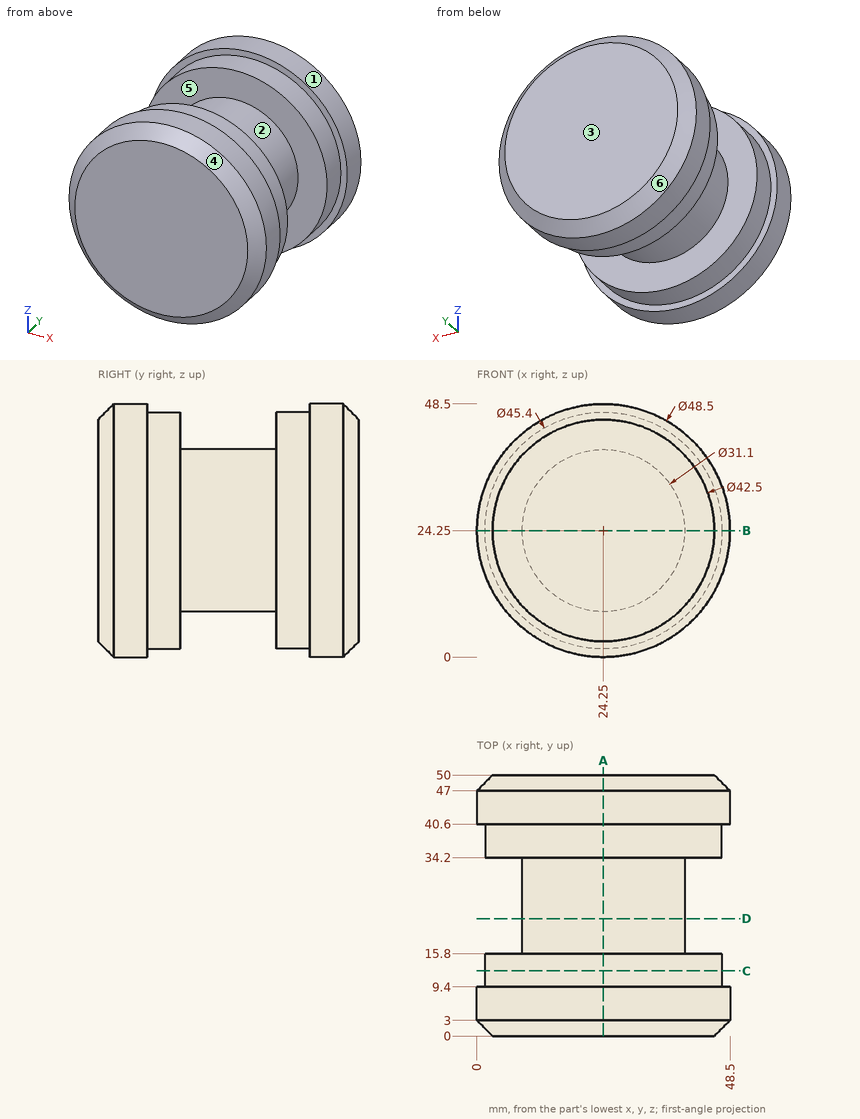
Answer from the drawing. Dimensions are ordinates in mm from the lowest x, y and z of the part. A direction names the side the tool comes from. Coordinates: 2 decimals unless noted, no trailing zeros. Write each loop counter-clockwise with the first axis right and the second up, starting at its lowest first coordinate (ties: lowest second). Pieces come first, ordered by that corner, then holes. Notation, with made-up numbers: (57.25, -14) -> (64.25, -14) arc R23 ccw to (64.25, 21) -> close; hole circle Ø11 at (-17, 40). An arc over 180 degrees is marked (long way). One line per question, with ' | ' between items.
1. Section A-A (x = 24.25) is taken. Determine the outline of the cut face in (y, z), and give its area (3 significant figures).
Verdict:
outline: (0, 3) -> (3, 0) -> (9.4, 0) -> (9.4, 1.55) -> (15.8, 1.55) -> (15.8, 8.7) -> (34.2, 8.7) -> (34.2, 1.55) -> (40.6, 1.55) -> (40.6, 0) -> (47, 0) -> (50, 3) -> (50, 45.5) -> (47, 48.5) -> (40.6, 48.5) -> (40.6, 46.95) -> (34.2, 46.95) -> (34.2, 39.8) -> (15.8, 39.8) -> (15.8, 46.95) -> (9.4, 46.95) -> (9.4, 48.5) -> (3, 48.5) -> (0, 45.5) -> close | area: 2,050 mm^2
2. Given pin 1 Ø2 at (y, z) = (39.5, 22) entering from +X; pin 2 Ø5 at (x, y) = (40.5, 10) entering from +Z; pin 3 Ø4 at (y, z) = (18.5, 31.5) entering from -X, each flat-ended and moving along its own axis, determine where each tip first touches the part or whether it passes through.
Verdict:
pin 1: stops at x = 46.92 | pin 2: stops at z = 44.17 | pin 3: stops at x = 9.61
3. Which of the six approach directions +Z, -Z, +X, -X, +Y, -Y give full straight-line access (tool end or side, diameter ignored) to the marked faces 5 and 6?
Verdict:
face 5: none | face 6: +Y
4. Section D-D (y = 22.5) is taken. Determine the outline of the cut face in (x, z), and give its area (3 significant figures).
Verdict:
outline: circle Ø31.1 at (24.25, 24.25) | area: 760 mm^2
5. Section C-C (y = 12.5) is taken. Determine the outline of the cut face in (x, z).
Verdict:
outline: circle Ø45.4 at (24.25, 24.25)
6. Straight lines are drawn through the part: line 1 (Y direction, x = 7.5, z = 36.5); line 2 (Y direction, x = 23.5, z = 46.5); line 3 (X direction, y = 41, z = 23.5). For each, find the intervals that lie inside material, in ascending order.
Verdict:
line 1: y = 0 to 15.8, 34.2 to 50 | line 2: y = 1.01 to 15.8, 34.2 to 48.99 | line 3: x = 0.01 to 48.49
7. Section B-B (z = 24.25) is taken. Determine the outline of the cut face in (x, y), and give its area (3 significant figures).
Verdict:
outline: (0, 3) -> (3, 0) -> (45.5, 0) -> (48.5, 3) -> (48.5, 9.4) -> (46.95, 9.4) -> (46.95, 15.8) -> (39.8, 15.8) -> (39.8, 34.2) -> (46.95, 34.2) -> (46.95, 40.6) -> (48.5, 40.6) -> (48.5, 47) -> (45.5, 50) -> (3, 50) -> (0, 47) -> (0, 40.6) -> (1.55, 40.6) -> (1.55, 34.2) -> (8.7, 34.2) -> (8.7, 15.8) -> (1.55, 15.8) -> (1.55, 9.4) -> (0, 9.4) -> close | area: 2,050 mm^2
8. For a pull along Y with two mould halves and no side action, classify the marked faces 1, 2, 3 and 4 as released by +Y, released by -Y, zero draft, split by the parting line, or undercut.
Verdict:
face 1: zero draft | face 2: undercut | face 3: released by +Y | face 4: released by -Y
